from build123d import *

# Parameters (mm, degrees)
BASE_FLANGE1_DEPTH = 3.0226
FILLET1_R          = 6.35
FILLET2_R          = 0.396875


# Sheet-metal steps are written as plain solids
with BuildPart() as part:
    # Sketch1 → Base-Flange1 (new body)
    with BuildSketch(Plane(origin=(0, 0, 0), x_dir=(0, 0, -1), z_dir=(1, 0, 0))):
        Polygon((0, -19.05), (0, -50.8), (8.466666667, -50.8), (25.4, 0), (0, 0), (-3.175, 0), (-3.175, -19.05), align=None)
    extrude(amount=-BASE_FLANGE1_DEPTH)

    # Fillet1
    fillet1_edges = [part.edges().sort_by_distance(p)[0] for p in [
        (-1.5113, 0, -25.4),
        (-1.5113, -50.8, -8.466666667),
    ]]
    fillet(fillet1_edges, radius=FILLET1_R)

    # Fillet2
    fillet2_edges = [part.edges().sort_by_distance(p)[0] for p in [
        (-1.5113, -50.8, 0),
        (-1.5113, -19.05, 0),
        (-1.5113, -19.05, 3.175),
        (-1.5113, 0, 3.175),
    ]]
    fillet(fillet2_edges, radius=FILLET2_R)


solid = part.part
Source: CAD feature listing. Evaluate the final solid. Frame: model axes, mm. A direction names the side the tool comes from. Round coordinates to 2 decimals unless told otherwise and drop trailing zeros. Write each loop counter-clockwise with the first axis right and the second up, starting at its lowest first coordinate (ties: lowest second). Pieces come first, ordered by that corner, then holes. Notation, with made-up numbers: M 32.5,78 L 84.5,78 A20 ccw 84.5,87 Z; hole C -27,64.5 d6. An arc over 180 degrees is marked long. One line per item, written item: value. Start each with the question number.
Item 1: Pin query (flat end, axial travel): pin 1 (1.5 mm diameter, centred on x = -1.5, y = -39, fed in from +Z); pin 2 (1.2 mm diameter, centred on x = -1.5, z = 2, fed in from -Y); pin 3 (1.5 mm diameter, centred on x = -2.5, y = -8, fed in from -Z). Return the tip coordinate at first contact, or that it passes through.
Item 2: Ray query, L1, parallel to Y at x = -0.4, z = 1.25; L2, parallel to Z at x = -2.3, y = -9 (3 decimals); L3, parallel to Z at x = -1.4, y = -31. Return the intervals inside material, ascending. Write a range as from..to.
Item 3: Section query B-B (z = -10.75). Return the cut outline in (x, y), plus the area to 3 significant figures.
Item 4: Section query A-A (x = -1.4). Return the cut outline in (y, z) (3 decimals), plus the area to 3 significant figures.
Item 5: Section query C-C (y = -39). Return the cut outline in (x, z), plus the area to 3 significant figures.
Item 6: Set-up query: faces 1 (the flat face through (-1, -19.05, 2)), 2 (the flat face through (-3.023, -19, -7)). Return all of +Z, -Z, +X, -X, +Y, -Y with unobstructed straight access to the full face (end or side cutting, diameter ignored); none if empty.
Result set:
1. pin 1: stops at z = 0
1. pin 2: stops at y = -19.05
1. pin 3: stops at z = -22.88
2. L1: y = -19.05..0
2. L2: z = -22.4..3.175
2. L3: z = -15.07..0
3. outline: M -3.02,-43.95 L 0,-43.95 L 0,0 L -3.02,0 Z
3. area: 133 mm²
4. outline: M -50.8,-3.89 A6.35 ccw -46.458,-9.914 L -8.358,-22.614 A6.35 ccw 0,-16.59 L 0,2.778 A0.397 ccw -0.397,3.175 L -18.653,3.175 A0.397 ccw -19.05,2.778 L -19.05,0.397 A0.397 cw -19.447,0 L -50.403,0 A0.397 ccw -50.8,-0.397 Z
4. area: 899 mm²
5. outline: M -3.02,-12.4 L 0,-12.4 L 0,0 L -3.02,0 Z
5. area: 37.5 mm²
6. face 1: +Z, +X, -X, -Y
6. face 2: +Z, -Z, -X, +Y, -Y
